Check sheet for the drawn part. Datum: minimum x, y, z corner. Units: mm. A direction names the side the tool comes from. Give positions to 0.01 mm unless a question says otherwise; leave off trailing zeros. Loops run counter-clockwise (first coordinate to the right, second up) from the corner with the lowest first, then second, coordinate; pieces in that order, holes last. Notation, with made-up numbers: (-3.5, -17.5) -> (15.5, -17.5) arc R19 ccw to (15.5, 18.5) -> close; hole circle Ø4 at (61, 57). An arc over 180 degrees is marked (long way). One line per question, with ' | ' between items.
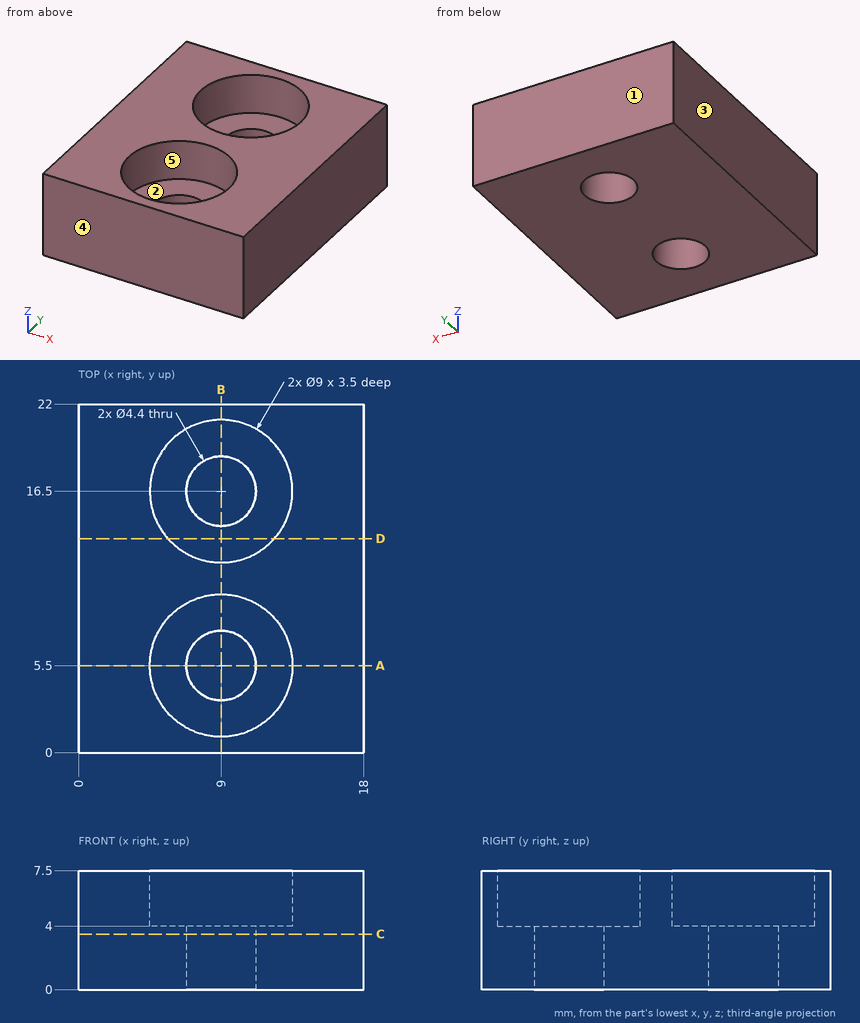
Item 1: Set-up check for the marked faces 4 and 5: record each of +Z, -Z, +X, -X, +Y, -Y from which the full face is reachable in a straight line by a thin tool's end or side.
Result:
face 4: +Z, -Z, +X, -X, -Y | face 5: +Z
Item 2: Sectioned sample at A-A (y = 5.5). Record the cut outline in (x, z), plus the area to 3 significant figures.
Result:
outline: (0, 0) -> (6.8, 0) -> (6.8, 4) -> (4.5, 4) -> (4.5, 7.5) -> (0, 7.5) -> close; (11.2, 0) -> (18, 0) -> (18, 7.5) -> (13.5, 7.5) -> (13.5, 4) -> (11.2, 4) -> close | area: 85.9 mm2
Item 3: Scan lines: probe 1 along Y at (x, z) = (9, 2.65); probe 2 along Y at (x, z) = (9, 5.05); probe 3 along X at (y, z) = (5.5, 2.85). Record each from-to range of solid material in increasing order.
Result:
probe 1: 0 to 3.3, 7.7 to 14.3, 18.7 to 22 | probe 2: 0 to 1, 10 to 12, 21 to 22 | probe 3: 0 to 6.8, 11.2 to 18
Item 4: Sectioned sample at C-C (z = 3.5). Record the cut outline in (x, y), plus the area to 3 significant figures.
Result:
outline: (0, 0) -> (18, 0) -> (18, 22) -> (0, 22) -> close; hole circle Ø4.4 at (9, 5.5); hole circle Ø4.4 at (9, 16.5) | area: 366 mm2
Item 5: Sectioned sample at B-B (x = 9). Record the cut outline in (y, z).
Result:
outline: (0, 0) -> (3.3, 0) -> (3.3, 4) -> (1, 4) -> (1, 7.5) -> (0, 7.5) -> close; (7.7, 0) -> (14.3, 0) -> (14.3, 4) -> (12, 4) -> (12, 7.5) -> (10, 7.5) -> (10, 4) -> (7.7, 4) -> close; (18.7, 0) -> (22, 0) -> (22, 7.5) -> (21, 7.5) -> (21, 4) -> (18.7, 4) -> close
Item 6: Release check for a two-part mould opening along X. For the marked faces 1, 2 and 3 record: pulls with the +X half, pulls with the -X half, needs draft (parallel to the pull), parting line crosses it, or undercut.
Result:
face 1: needs draft | face 2: undercut | face 3: pulls with the -X half
Item 7: Depth check by flat-ended pin: pin 1 Ø10 at (x, y) = (6.5, 10) entering from -Z; pin 2 Ø2.5 at (x, y) = (11, 15.5) entering from +Z. Enter the tip coordinate at first touch or a pass-through.
Result:
pin 1: z = 0 | pin 2: z = 4
Item 8: Sectioned sample at D-D (y = 13.5). Record the cut outline in (x, z), plus the area to 3 significant figures.
Result:
outline: (0, 0) -> (18, 0) -> (18, 7.5) -> (12.35, 7.5) -> (12.35, 4) -> (5.65, 4) -> (5.65, 7.5) -> (0, 7.5) -> close | area: 112 mm2
